```python
from build123d import *

# Parameters (mm, degrees)
BOSS_EXTRUDE1_DEPTH     = 1
SKETCH2_R               = 1.475
BOSS_EXTRUDE2_DEPTH     = 14
SKETCH3_R               = 1.8
BOSS_EXTRUDE3_DEPTH     = 1
SKETCH4_W               = 2
SKETCH4_H               = 17
BOSS_EXTRUDE4_DEPTH     = 12
SKETCH5_W               = 18
SKETCH5_H               = 2
BOSS_EXTRUDE5_DEPTH     = 12
SKETCH6_W               = 13
SKETCH6_H               = 2
BOSS_EXTRUDE6_DEPTH     = 5
BOSS_EXTRUDE7_DEPTH     = 12
CUT_EXTRUDE1_DEPTH      = 24.366642891
SKETCH9_W               = 2.937742252
SKETCH9_H               = 8
CUT_EXTRUDE2_DEPTH      = 12
CUT_EXTRUDE11_START     = -12
SKETCH21_R              = 10.5
SKETCH21_R_2            = 1.8
CUT_EXTRUDE11_DEPTH     = 12
SKETCH10_W              = 32
SKETCH10_H              = 2
BOSS_EXTRUDE8_DEPTH     = 7
FILLET1_R               = 0.5
SKETCH11_R              = 0.625
BOSS_EXTRUDE9_DEPTH     = 2
SKETCH14_W              = 2
SKETCH14_H              = 2
CUT_EXTRUDE5_DEPTH      = 28.874719859
SKETCH12_R              = 0.675
CUT_EXTRUDE3_DEPTH      = 2.5
CUT_EXTRUDE6_DEPTH      = 2
FILLET2_R               = 0.5
FILLET3_R               = 0.5
FILLET4_R               = 2
CUT_EXTRUDE7_DEPTH      = 28.221315288
CUT_EXTRUDE7_DEPTH_BACK = 1
SKETCH19_R              = 0.625
CUT_EXTRUDE9_DEPTH      = 2


with BuildPart() as part:
    # Sketch1 → Boss-Extrude1 (new body)
    with BuildSketch(Plane.XY):
        Polygon((-11, 6), (-11, 11), (11, 11), (11, 6), (11, -6), (-11, -6), align=None)
    extrude(amount=BOSS_EXTRUDE1_DEPTH)

    # Sketch2 → Boss-Extrude2 (add)
    with BuildSketch(Plane(origin=(0, 0, 0), x_dir=(-1, 0, 0), z_dir=(0, 0, -1))):
        with Locations(Location((0, 0, 0), (0, 0, 180))):
            Circle(SKETCH2_R)
    extrude(amount=BOSS_EXTRUDE2_DEPTH)

    # Sketch3 → Boss-Extrude3 (add)
    with BuildSketch(Plane(origin=(0, 0, 0), x_dir=(-1, 0, 0), z_dir=(0, 0, -1))):
        with Locations(Location((0, 0, 0), (0, 0, 180))):
            Circle(SKETCH3_R)
    extrude(amount=BOSS_EXTRUDE3_DEPTH)

    # Sketch4 → Boss-Extrude4 (add)
    with BuildSketch(Plane(origin=(0, 0, 0), x_dir=(-1, 0, 0), z_dir=(0, 0, -1))):
        with Locations((10, 2.5)):
            Rectangle(SKETCH4_W, SKETCH4_H)
        with Locations((-10, 2.5)):
            Rectangle(SKETCH4_W, SKETCH4_H)
    extrude(amount=BOSS_EXTRUDE4_DEPTH)

    # Sketch5 → Boss-Extrude5 (add)
    with BuildSketch(Plane(origin=(0, 0, 0), x_dir=(-1, 0, 0), z_dir=(0, 0, -1))):
        with Locations((0, 10)):
            Rectangle(SKETCH5_W, SKETCH5_H)
    extrude(amount=BOSS_EXTRUDE5_DEPTH)

    # Sketch6 → Boss-Extrude6 (add)
    with BuildSketch(Plane(origin=(11, 0, 0), x_dir=(0, 0, -1), z_dir=(1, 0, 0))):
        with Locations((5.5, -5)):
            Rectangle(SKETCH6_W, SKETCH6_H)
        with Locations((5.5, 5)):
            Rectangle(SKETCH6_W, SKETCH6_H)
    boss_extrude6 = extrude(amount=BOSS_EXTRUDE6_DEPTH)

    # Mirror1: Boss-Extrude6 across plane
    add(boss_extrude6.mirror(Plane(origin=(0, 0, 0), x_dir=(0, 0, 1), z_dir=(1, 0, 0))))

    # Sketch7 → Boss-Extrude7 (add)
    with BuildSketch(Plane(origin=(0, 0, -12), x_dir=(-1, 0, 0), z_dir=(0, 0, -1))):
        with BuildLine():
            ThreePointArc((-6.708203932, -6), (-8.407551231, -3.211398808), (-9, 0))
            Line((-9, 0), (-9, -6))
            Line((-9, -6), (-6.708203932, -6))
        make_face()
        with BuildLine():
            Line((-9, 9), (-9, 0))
            ThreePointArc((-9, 0), (-6.363961031, 6.363961031), (0, 9))
            Line((0, 9), (-9, 9))
        make_face()
    boss_extrude7 = extrude(amount=-BOSS_EXTRUDE7_DEPTH)

    # Sketch8 → Cut-Extrude1 (cut, through all)
    with BuildSketch(Plane(origin=(0, 0, -12), x_dir=(-1, 0, 0), z_dir=(0, 0, -1))):
        with BuildLine():
            Line((-11, 4), (-9.16515139, 4))
            ThreePointArc((-9.16515139, 4), (-10, 0), (-9.16515139, -4))
            Line((-9.16515139, -4), (-11, -4))
            Line((-11, -4), (-11, 4))
        make_face()
    cut_extrude1 = extrude(amount=-CUT_EXTRUDE1_DEPTH, mode=Mode.SUBTRACT)

    # Sketch9 → Cut-Extrude2 (cut)
    with BuildSketch(Plane(origin=(0, 0, -12), x_dir=(-1, 0, 0), z_dir=(0, 0, -1))):
        with Locations((-9.531128874, 0)):
            Rectangle(SKETCH9_W, SKETCH9_H)
    cut_extrude2 = extrude(amount=-CUT_EXTRUDE2_DEPTH, mode=Mode.SUBTRACT)

    # Mirror2: Boss-Extrude7, Cut-Extrude1, Cut-Extrude2 across plane
    add(boss_extrude7.mirror(Plane(origin=(0, 0, 0), x_dir=(0, 0, 1), z_dir=(1, 0, 0))))
    add(cut_extrude1.mirror(Plane(origin=(0, 0, 0), x_dir=(0, 0, 1), z_dir=(1, 0, 0))), mode=Mode.SUBTRACT)
    add(cut_extrude2.mirror(Plane(origin=(0, 0, 0), x_dir=(0, 0, 1), z_dir=(1, 0, 0))), mode=Mode.SUBTRACT)

    # Sketch21 → Cut-Extrude11 (cut)
    with BuildSketch(Plane(origin=(0, 0, -12), x_dir=(-1, 0, 0), z_dir=(0, 0, -1)).offset(CUT_EXTRUDE11_START)):
        Circle(SKETCH21_R)
        with Locations(Location((0, 0, 0), (0, 0, 180))):
            Circle(SKETCH21_R_2, mode=Mode.SUBTRACT)
    extrude(amount=CUT_EXTRUDE11_DEPTH, mode=Mode.SUBTRACT)

    # Sketch10 → Boss-Extrude8 (add)
    with BuildSketch(Plane.XY.offset(1)):
        with Locations((0, -5)):
            Rectangle(SKETCH10_W, SKETCH10_H)
        with Locations((0, 5)):
            Rectangle(SKETCH10_W, SKETCH10_H)
    extrude(amount=BOSS_EXTRUDE8_DEPTH)

    # Fillet1
    fillet1_edges = [part.edges().sort_by_distance(p)[0] for p in [
        (10, 0, 1),
        (-10, 0, 1),
    ]]
    fillet(fillet1_edges, radius=FILLET1_R)

    # Sketch11 → Boss-Extrude9 (add)
    with BuildSketch(Plane(origin=(0, 0, -12), x_dir=(-1, 0, 0), z_dir=(0, 0, -1))):
        with Locations(Location((-13, -5, 0), (0, 0, 180))):
            Circle(SKETCH11_R)
    boss_extrude9 = extrude(amount=BOSS_EXTRUDE9_DEPTH)

    # Sketch14 → Cut-Extrude5 (cut, through all)
    with BuildSketch(Plane(origin=(0, 0, -12), x_dir=(-1, 0, 0), z_dir=(0, 0, -1))):
        with Locations((10, 7)):
            Rectangle(SKETCH14_W, SKETCH14_H)
        with Locations((-10, 7)):
            Rectangle(SKETCH14_W, SKETCH14_H)
    extrude(amount=-CUT_EXTRUDE5_DEPTH, mode=Mode.SUBTRACT)

    # Sketch12 → Cut-Extrude3 (cut)
    with BuildSketch(Plane(origin=(0, 0, -12), x_dir=(-1, 0, 0), z_dir=(0, 0, -1))):
        with Locations((13, -5)):
            Circle(SKETCH12_R)
    cut_extrude3 = extrude(amount=-CUT_EXTRUDE3_DEPTH, mode=Mode.SUBTRACT)

    # Sketch16 → Cut-Extrude6 (cut)
    with BuildSketch(Plane(origin=(0, 6, 0), x_dir=(1, 0, 0), z_dir=(0, 1, 0))):
        with BuildLine():
            Line((-9, 0), (-9, -1))
            ThreePointArc((-9, -1), (-8.75, -0.5), (-9, 0))
        make_face()
    cut_extrude6 = extrude(amount=CUT_EXTRUDE6_DEPTH, mode=Mode.SUBTRACT)

    # Mirror3: Boss-Extrude9, Cut-Extrude3 across plane
    add(boss_extrude9.mirror(Plane.ZX))
    add(cut_extrude3.mirror(Plane.ZX), mode=Mode.SUBTRACT)

    # Mirror4: Cut-Extrude6 across plane
    add(cut_extrude6.mirror(Plane(origin=(0, 0, 0), x_dir=(0, 0, 1), z_dir=(1, 0, 0))), mode=Mode.SUBTRACT)

    # Fillet2
    fillet2_edges = [part.edges().sort_by_distance(p)[0] for p in [
        (12.375, -5, -12),
        (12.375, 5, -12),
    ]]
    fillet(fillet2_edges, radius=FILLET2_R)

    # Fillet3
    # the kernel refuses this fillet: 0.5 mm, written as the material it takes off along each edge
    with BuildSketch(Plane(origin=(-13, -5, -12), x_dir=(-1, 0, 0), z_dir=(0, -1, 0))) as fillet3_piece_1:
        with BuildLine():
            CenterArc((0.675 + FILLET3_R, -FILLET3_R), FILLET3_R, 90, 90)
            Line((0.675, -FILLET3_R), (0.675, 0))
            Line((0.675, 0), (0.675 + FILLET3_R, 0))
        make_face()
    revolve(axis=Axis((-13, -5, -12), (0, 0, -1)), mode=Mode.SUBTRACT)
    with BuildSketch(Plane(origin=(-13, 5, -12), x_dir=(-1, 0, 0), z_dir=(0, 1, 0))) as fillet3_piece_2:
        with BuildLine():
            CenterArc((0.675 + FILLET3_R, FILLET3_R), FILLET3_R, 180, 90)
            Line((0.675, FILLET3_R), (0.675, 0))
            Line((0.675, 0), (0.675 + FILLET3_R, 0))
        make_face()
    revolve(axis=Axis((-13, 5, -12), (0, 0, 1)), mode=Mode.SUBTRACT)

    # Fillet4
    fillet4_edges = [part.edges().sort_by_distance(p)[0] for p in [
        (16, -5, 8),
        (-16, -5, 8),
        (-16, 5, 8),
        (16, 5, 8),
    ]]
    fillet(fillet4_edges, radius=FILLET4_R)

    # Sketch17 → Cut-Extrude7 (cut, two sides: drawn at the far end of the back side and taken through both)
    with BuildSketch(Plane.XZ.offset(6).offset(-CUT_EXTRUDE7_DEPTH_BACK)):
        with BuildLine():
            Line((-16, 6), (-16, -12))
            Line((-16, -12), (-14.5, -12))
            Line((-14.5, -12), (-14.5, 6))
            ThreePointArc((-14.5, 6), (-14.353553391, 6.353553391), (-14, 6.5))
            Line((-14, 6.5), (14, 6.5))
            ThreePointArc((14, 6.5), (14.353553391, 6.353553391), (14.5, 6))
            Line((14.5, 6), (14.5, -12))
            Line((14.5, -12), (16, -12))
            Line((16, -12), (16, 6))
            ThreePointArc((16, 6), (15.414213562, 7.414213562), (14, 8))
            Line((14, 8), (-14, 8))
            ThreePointArc((-14, 8), (-15.414213562, 7.414213562), (-16, 6))
        make_face()
    extrude(amount=CUT_EXTRUDE7_DEPTH + CUT_EXTRUDE7_DEPTH_BACK, mode=Mode.SUBTRACT)

    # Sketch19 → Cut-Extrude9 (cut)
    with BuildSketch(Plane(origin=(0, 6, 0), x_dir=(1, 0, 0), z_dir=(0, 1, 0))):
        with Locations(Location((0, -1.625, 0), (0, 0, 90))):
            Circle(SKETCH19_R)
        with Locations(Location((0, -6.625, 0), (0, 0, 270))):
            Circle(SKETCH19_R)
    extrude(amount=-CUT_EXTRUDE9_DEPTH, mode=Mode.SUBTRACT)


solid = part.part
```
Model file for the job. Use its own axes, mm. A direction names the side the tool comes from. Coordinates: 2 decimals unless noted, no trailing zeros. Loops run counter-clockwise (first coordinate to the right, second up) from the corner with the lowest first, then second, coordinate; pieces in that order, holes last. Notation, with made-up numbers: (-31, 80.5) - (-23, 80.5) arc R36 cw to (-23, 118.5) - close; hole circle Ø2 at (27, 20). An arc over 180 degrees is marked (long way). Answer as a JSON object with one key per item and string values. Group by question number.
(1) Cut at D-D (x = -13). Give the cut face in (y, z) (3 decimals).
(2) Cut at C-C (y = 0). Give the cut face in (x, z) (3 decimals).
(3) Cut at B-B (z = 4.25). Give the cut face in (x, y), then the cut area to 3 significant figures.
(4) Cut at A-A (z = -8.5). Give the cut face in (x, y) (3 decimals).
(5) Probe line 1 along Y through (x, z) = (-13, -10.15) (3 decimals); line 2 along Y through (x, z) = (10, -4.5); line 3 along Y through (x, z) = (-11.5, -6). List the from-to ranges inside material, lowest first.
(6) Flat gauge pins, fed straight in: pin 1 (1.5 mm diameter, centred on x = -3, y = 9.5, fed in from +Z); pin 2 (8 mm diameter, centred on x = -10.5, y = 6.5, fed in from -Z); pin 3 (1.5 mm diameter, centred on y = 9.5, z = -4, fed in from +X). Where does each tip first touch, or does it go through?
(7) Tool access for faces 4 (the face through (-14.8, -4.8, -12)), 5 (the face through (8.75, 6.99, 0.51)), 6 (the face through (11, 9, -6)), 7 (the face through (9, 7, -6)), 8 (the face through (1.717, -0.541, -0.493)): list every direction of +Z, -Z, +X, -X, +Y, -Y with a clear straight run to the whole face (end or side of a thin tool).
(8) Two-plate mould, pull along X, no slides. Class faces 1 (the face through (-8.75, 6.99, 0.51)), 2 (the face through (14.8, -4.8, -12)), 3 (the face through (-13.36, -4.43, -10.51)): released by +X, released by -X, zero draft, split by the parting line, or undercut.
Geometry says:
{
 "1": {"outline": "(-6, -11.968) arc R0.5 ccw to (-5.675, -11.5) - (-5.675, -9.5) - (-4.325, -9.5) - (-4.325, -11.5) arc R0.5 ccw to (-4, -11.968) - (-4, 8) - (-5, 8) - (-5, 6.5) - (-6, 6.5) - close; (4, -11.968) arc R0.5 ccw to (4.325, -11.5) - (4.325, -9.5) - (5.675, -9.5) - (5.675, -11.5) arc R0.5 ccw to (6, -11.968) - (6, 8) - (4, 8) - close"},
 "2": {"outline": "(-10, 0) - (-1.8, 0) - (-1.8, -1) - (-1.475, -1) - (-1.475, -14) - (1.475, -14) - (1.475, -1) - (1.8, -1) - (1.8, 0) - (10, 0) - (10, 0.5) arc R0.5 ccw to (9.5, 1) - (-9.5, 1) arc R0.5 ccw to (-10, 0.5) - close"},
 "3": {"outline": "(-16, -5) - (-14.5, -5) - (-14.5, -6) - (14.5, -6) - (14.5, -5) - (16, -5) - (16, -4) - (-16, -4) - close; (-16, 4) - (16, 4) - (16, 6) - (-16, 6) - close", "area": "125 mm^2"},
 "4": {"outline": "(-16, -5) - (-14.5, -5) - (-14.5, -6) - (-8.617, -6) arc R10.5 cw to (-9.708, -4) - (-16, -4) - close; (-16, 4) - (-9.708, 4) arc R10.5 cw to (9.708, 4) - (16, 4) - (16, 6) - (9, 6) - (9, 8) - (11, 8) - (11, 11) - (-11, 11) - (-11, 8) - (-9, 8) - (-9, 6) - (-16, 6) - close; circle Ø2.95 at (0, 0); (8.617, -6) - (14.5, -6) - (14.5, -5) - (16, -5) - (16, -4) - (9.708, -4) arc R10.5 cw to start"},
 "5": {"line 1": "y = -6 to -5.675, -4.325 to -4, 4 to 4.325, 5.675 to 6", "line 2": "y = -6 to -4, 4 to 6, 8 to 11", "line 3": "y = -6 to -4, 4 to 6"},
 "6": {"pin 1": "stops at z = 1", "pin 2": "stops at z = -12", "pin 3": "stops at x = 11"},
 "7": {"face 4": "-Z, -X, +Y, -Y", "face 5": "+X", "face 6": "+Z, -Z, +X, +Y", "face 7": "+Z, -Z, +X", "face 8": "-Z"},
 "8": {"face 1": "released by -X", "face 2": "zero draft", "face 3": "undercut"}
}
